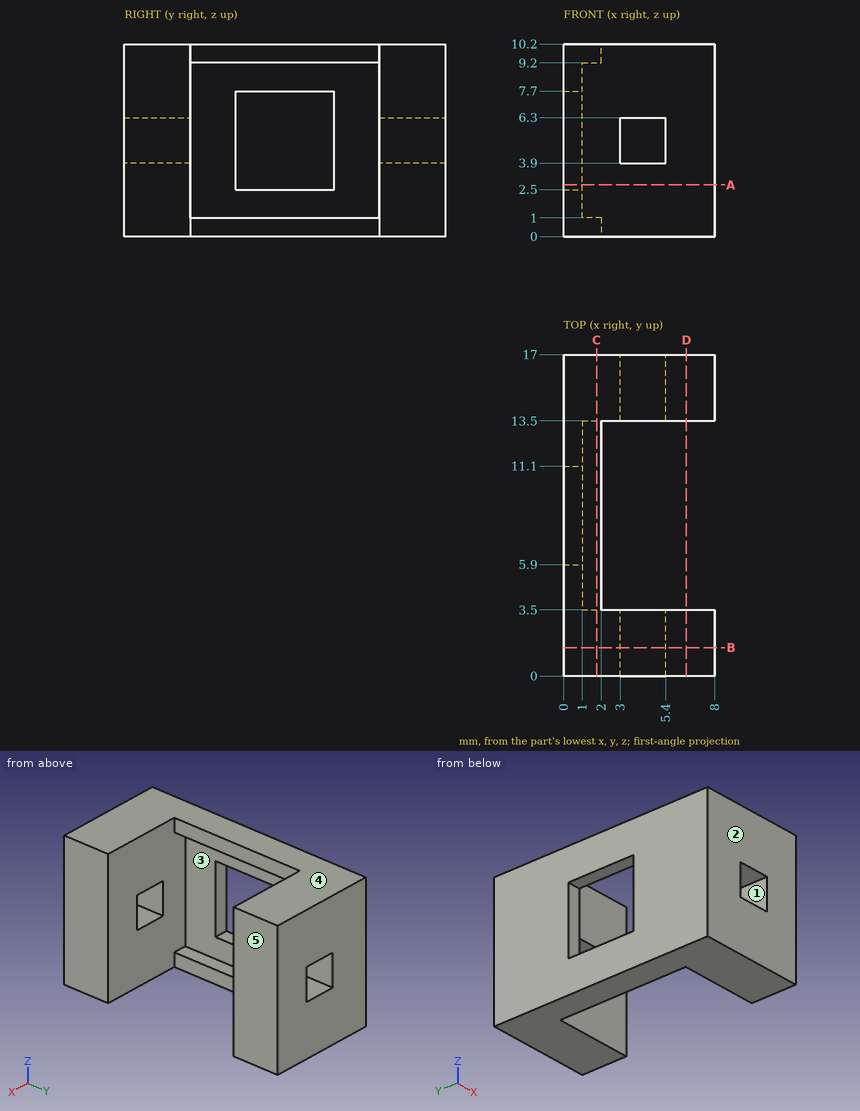
The drawing under review shows one solid part. Ordinate dimensions are in mm from its lowest x, y, z. A direction names the side the tool comes from. Give positions to 0.01 mm unless a question says otherwise; leave off trailing zeros. Order: outer loops, then holes, each group sorted by start corner. A loop starts at its lowest first (then second) coordinate and runs counter-clockwise, first axis right, second up. Notation, with made-up numbers: M 81.25,85.25 L 108.25,85.25 A20 ccw 108.25,93.25 Z; hole C 46,-22.5 d6. An arc over 180 degrees is marked long. Answer in a Markdown table with one row per item. Add a question column.
1. For pin 1 Ø2 at (x, y) = (6, 12) entering from +Z, flat-tipped, find the tip position at first contact; note if it passes through.
2. To check wall thickness, follow line 1 along Y through (x, z) = (4.5, 9); line 2 along X through (y, z) = (2.25, 6.25); line 3 along Z through (x, y) = (1.5, 10.75). State the ranges of each line that lie inside material, in increasing order.
3. Mouldability with a two-part tool opening along Z and no side actions: class the marked faces 3, 4 and 5 as released by +Z, released by -Z, zero draft, split by the parting line, or undercut.
4. Add section A-A on z = 2.75. State the section outline as (x, y) points.
5. Add section C-C on x = 1.75. State the section outline as (y, z) points.
6. Machinability: for the marked faces 1 and 2, which of the approach directions +Z, -Z, +X, -X, +Y, -Y give a long, thin tool a straight path to every point of the face, cutting with its end or side? Answer none if there is none.
7. Add section B-B on y = 1.5. State the section outline as (x, z) points.
8. Add section D-D on x = 6.5. State the section outline as (y, z) points.
The answers:
| question | item | result |
|---|---|---|
| 1 | pin 1 | through |
| 2 | line 1 | 0 to 3.5, 13.5 to 17 |
| 2 | line 2 | 0 to 3, 5.4 to 8 |
| 2 | line 3 | 0 to 1, 9.2 to 10.2 |
| 3 | face 3 | undercut |
| 3 | face 4 | released by +Z |
| 3 | face 5 | zero draft |
| 4 | outline | M 0,0 L 8,0 L 8,3.5 L 1,3.5 L 1,5.9 L 0,5.9 Z; M 0,11.1 L 1,11.1 L 1,13.5 L 8,13.5 L 8,17 L 0,17 Z |
| 5 | outline | M 0,0 L 17,0 L 17,10.2 L 0,10.2 Z; hole M 3.5,1 L 13.5,1 L 13.5,9.2 L 3.5,9.2 Z |
| 6 | face 1 | +Y, -Y |
| 6 | face 2 | +Z, -Z, +X, -X, -Y |
| 7 | outline | M 0,0 L 8,0 L 8,10.2 L 0,10.2 Z; hole M 3,3.9 L 5.4,3.9 L 5.4,6.3 L 3,6.3 Z |
| 8 | outline | M 0,0 L 3.5,0 L 3.5,10.2 L 0,10.2 Z; M 13.5,0 L 17,0 L 17,10.2 L 13.5,10.2 Z |
